Part model, mm, in its own coordinate system. A direction names the side the tool comes from. Round coordinates to 2 decimals unless told otherwise and drop trailing zeros. Loops run counter-clockwise (first coordinate to the right, second up) from the corner with the lowest first, then second, coordinate; pieces in that order, holes last. Notation, with made-up numbers: (-25.75, 8.5) -> (-0.75, 8.5) arc R25 cw to (-0.75, 22.5) -> close; hole circle Ø8 at (24, 24.5). An arc over 180 degrees is marked (long way). Answer as CSV lines item,"result".
from build123d import *

# Parameters (mm, degrees)
SALIENTE_EXTRUIR1_DEPTH = 33
CROQUIS2_W              = 6
CROQUIS2_H              = 3
SALIENTE_EXTRUIR2_DEPTH = 6


with BuildPart() as part:
    # Croquis1 → Saliente-Extruir1 (new, symmetric)
    with BuildSketch(Plane(origin=(0, 0, 0), x_dir=(1, 0, 0), z_dir=(0, 1, 0))):
        Polygon((-3.06, 6.21), (5.94, 6.21), (5.94, -2.79), (2.94, -2.79), (2.94, 3.21), (-3.06, 3.21), align=None)
    extrude(amount=SALIENTE_EXTRUIR1_DEPTH, both=True)

    # Croquis2 → Saliente-Extruir2 (add, through all)
    with BuildSketch(Plane.XY.offset(-3.21)):
        with Locations((-0.06, 31.5)):
            Rectangle(CROQUIS2_W, CROQUIS2_H)
    saliente_extruir2 = extrude(amount=SALIENTE_EXTRUIR2_DEPTH)

    # Simetría1: Saliente-Extruir2 across plane
    add(saliente_extruir2.mirror(Plane.ZX))


solid = part.part
Q1. Two-plate mould, pull along Y, no slides. Class faces 3 (the face through (0, -30, 0)), 4 (the face through (1, 33, -2)), 5 (the face through (0, 0, -3.21)), 6 (the face through (4, 0, 2.79)): pulls with the +Y half, pulls with the -Y half, needs draft (parallel to the pull), parting line crosses it, or undercut.
Geometry results:
face 3,"undercut"
face 4,"pulls with the +Y half"
face 5,"undercut"
face 6,"needs draft"
Q2. Which spindle directions (+Z, -Z, +X, -X, +Y, -Y) get a long thin tool onto all of the face, cutting with end or side? Do faces 1 (the face through (2.94, 0, 0)), 2 (the face through (1, -33, -2)). Say none if no direction does.
Geometry results:
face 1,"+Z, -X"
face 2,"+Z, -Z, +X, -X, -Y"
Q3. Saw through at B-B, the plane z = 0. Write the cut outline in (x, y), then the cut area to 3 significant figures.
Geometry results:
outline,"(-3.06, -33) -> (5.94, -33) -> (5.94, 33) -> (-3.06, 33) -> (-3.06, 30) -> (2.94, 30) -> (2.94, -30) -> (-3.06, -30) -> close"
area,"234 mm2"
Q4. Drill centre lines: line 1 along Y through (x, z) = (-1.75, -1.25); line 2 along X through (y, z) = (-19, -0.5); line 3 along Z through (x, y) = (-2, 27). Where is each one in solid material? Low to high.
Geometry results:
line 1,"-33 to -30, 30 to 33"
line 2,"2.94 to 5.94"
line 3,"-6.21 to -3.21"
Q5. Saw through at A-A, the plane x = 2. Write the cut outline in (y, z), then the cut area to 3 significant figures.
Geometry results:
outline,"(-33, -6.21) -> (33, -6.21) -> (33, 2.79) -> (30, 2.79) -> (30, -3.21) -> (-30, -3.21) -> (-30, 2.79) -> (-33, 2.79) -> close"
area,"234 mm2"
Q6. Saw through at C-C, the plane y = -14. Write the cut outline in (x, z).
Geometry results:
outline,"(-3.06, -6.21) -> (5.94, -6.21) -> (5.94, 2.79) -> (2.94, 2.79) -> (2.94, -3.21) -> (-3.06, -3.21) -> close"
Q7. Drop a flat-ended pin along its axis: P1, Ø1.5, axis at y = -8.5, z = -1, coming from the -X side. Give the stop position or say it passes through.
Geometry results:
P1,"x = 2.94"
